```python
from build123d import *

# Parameters (mm, degrees)
MODEL_R             = 2.9
MODEL_R_2           = 3
MODEL_R_3           = 1.95
MODEL_R_4           = 4.665
MODEL_W             = 19.6
MODEL_H             = 4.75
BOSS_EXTRUDE1_DEPTH = 5.15


with BuildPart() as part:
    # Model → Boss-Extrude1 (new body)
    with BuildSketch(Plane.XY):
        with BuildLine():
            Line((43.819984585, 81.048439688), (48.280015415, 78.473439688))
            Line((48.280015415, 78.473439688), (57.214943747, 93.949189523))
            ThreePointArc((57.214943747, 93.949189523), (60.358438208, 91.961181686), (63.432925851, 89.868036131))
            Line((63.432925851, 89.868036131), (56.520818931, 77.895915758))
            Line((56.520818931, 77.895915758), (60.020818931, 71.833737931))
            Line((60.020818931, 71.833737931), (72.810336239, 79.217769192))
            Line((72.810336239, 79.217769192), (79.758802159, 67.182673184))
            ThreePointArc((79.758802159, 67.182673184), (87.004437854, 62.632864027), (87.321870319, 54.083054869))
            Line((87.321870319, 54.083054869), (92.810336239, 44.57675304))
            Line((92.810336239, 44.57675304), (80.020818931, 37.19272178))
            Line((80.020818931, 37.19272178), (95.720818931, 9.999524101))
            Line((95.720818931, 9.999524101), (109.544554943, 9.999524101))
            ThreePointArc((109.544554943, 9.999524101), (109.819966834, 6.290857214), (109.969856665, 2.575))
            Line((109.969856665, 2.575), (92.1, 2.575))
            Line((92.1, 2.575), (92.1, -2.575))
            Line((92.1, -2.575), (109.969856665, -2.575))
            ThreePointArc((109.969856665, -2.575), (109.819947856, -6.291188516), (109.544494609, -10.000185045))
            Line((109.544494609, -10.000185045), (95.720280769, -10.000185045))
            Line((95.720280769, -10.000185045), (56.520280769, -77.896576702))
            Line((56.520280769, -77.896576702), (63.432272389, -89.86849737))
            ThreePointArc((63.432272389, -89.86849737), (60.358103868, -91.961401128), (57.214943747, -93.949189523))
            Line((57.214943747, -93.949189523), (48.280015415, -78.473439688))
            Line((48.280015415, -78.473439688), (43.819984585, -81.048439688))
            Line((43.819984585, -81.048439688), (52.754912918, -96.524189523))
            ThreePointArc((52.754912918, -96.524189523), (49.461727838, -98.252417168), (46.112001713, -99.868329805))
            Line((46.112001713, -99.868329805), (39.2, -87.896391657))
            Line((39.2, -87.896391657), (32.2, -87.896391657))
            Line((32.2, -87.896391657), (32.2, -102.664454178))
            Line((32.2, -102.664454178), (18.303068161, -102.664454178))
            ThreePointArc((18.303068161, -102.664454178), (10.74, -106.664454178), (3.17693184, -102.664454178))
            Line((3.17693184, -102.664454178), (-7.8, -102.664454178))
            Line((-7.8, -102.664454178), (-7.8, -87.896391657))
            Line((-7.8, -87.896391657), (-39.2, -87.896391657))
            Line((-39.2, -87.896391657), (-46.112001713, -99.868329805))
            ThreePointArc((-46.112001713, -99.868329805), (-49.461727838, -98.252417168), (-52.754912918, -96.524189523))
            Line((-52.754912918, -96.524189523), (-43.819984585, -81.048439689))
            Line((-43.819984585, -81.048439689), (-48.280015415, -78.473439689))
            Line((-48.280015415, -78.473439689), (-57.214943747, -93.949189523))
            ThreePointArc((-57.214943747, -93.949189523), (-60.358012455, -91.961461126), (-63.432093724, -89.868623478))
            Line((-63.432093724, -89.868623478), (-56.52019722, -77.896867556))
            Line((-56.52019722, -77.896867556), (-60.02019722, -71.834689729))
            Line((-60.02019722, -71.834689729), (-72.809714528, -79.218720989))
            Line((-72.809714528, -79.218720989), (-79.758180447, -67.183624982))
            ThreePointArc((-79.758180447, -67.183624982), (-87.003816143, -62.633815824), (-87.321248608, -54.084006667))
            Line((-87.321248608, -54.084006667), (-92.809714528, -44.577704838))
            Line((-92.809714528, -44.577704838), (-80.02019722, -37.193673578))
            Line((-80.02019722, -37.193673578), (-95.72019722, -10.000475899))
            Line((-95.72019722, -10.000475899), (-109.544468057, -10.000475899))
            ThreePointArc((-109.544468057, -10.000475899), (-109.819939504, -6.291334309), (-109.969856665, -2.575))
            Line((-109.969856665, -2.575), (-92.1, -2.575))
            Line((-92.1, -2.575), (-92.1, 2.575))
            Line((-92.1, 2.575), (-109.969856665, 2.575))
            ThreePointArc((-109.969856665, 2.575), (-109.819958483, 6.291003006), (-109.544528393, 9.999814955))
            Line((-109.544528393, 9.999814955), (-95.720735382, 9.999814955))
            Line((-95.720735382, 9.999814955), (-56.520735382, 77.896206612))
            Line((-56.520735382, 77.896206612), (-63.432747187, 89.86816224))
            ThreePointArc((-63.432747187, 89.86816224), (-60.358346795, 91.961241684), (-57.214943747, 93.949189523))
            Line((-57.214943747, 93.949189523), (-48.280015415, 78.473439689))
            Line((-48.280015415, 78.473439689), (-43.819984585, 81.048439689))
            Line((-43.819984585, 81.048439689), (-52.754912918, 96.524189523))
            ThreePointArc((-52.754912918, 96.524189523), (-49.461727838, 98.252417168), (-46.112001713, 99.868329805))
            Line((-46.112001713, 99.868329805), (-39.2, 87.896391657))
            Line((-39.2, 87.896391657), (-32.2, 87.896391657))
            Line((-32.2, 87.896391657), (-32.2, 102.664454178))
            Line((-32.2, 102.664454178), (-18.30306816, 102.664454178))
            ThreePointArc((-18.30306816, 102.664454178), (-10.74, 106.664454178), (-3.176931839, 102.664454178))
            Line((-3.176931839, 102.664454178), (7.8, 102.664454178))
            Line((7.8, 102.664454178), (7.8, 87.896391657))
            Line((7.8, 87.896391657), (39.2, 87.896391657))
            Line((39.2, 87.896391657), (46.112001713, 99.868329805))
            ThreePointArc((46.112001713, 99.868329805), (49.461727838, 98.252417168), (52.754912918, 96.524189523))
            Line((52.754912918, 96.524189523), (43.819984585, 81.048439688))
        make_face()
        with Locations((-63, 0)):
            Circle(MODEL_R, mode=Mode.SUBTRACT)
        with Locations((-31.5, -54.559600438)):
            Circle(MODEL_R, mode=Mode.SUBTRACT)
        with Locations((31.5, -54.559600438)):
            Circle(MODEL_R, mode=Mode.SUBTRACT)
        with Locations((63, 0)):
            Circle(MODEL_R, mode=Mode.SUBTRACT)
        with Locations((31.5, 54.559600438)):
            Circle(MODEL_R, mode=Mode.SUBTRACT)
        with Locations((-31.5, 54.559600438)):
            Circle(MODEL_R_2, mode=Mode.SUBTRACT)
        with Locations((-79.079683698, -58.058815824)):
            Circle(MODEL_R_3, mode=Mode.SUBTRACT)
        with Locations((79.08030541, 58.057864027)):
            Circle(MODEL_R_3, mode=Mode.SUBTRACT)
        Circle(MODEL_R_4, mode=Mode.SUBTRACT)
        with Locations((-10.74, 97.514454178)):
            Circle(MODEL_R_3, mode=Mode.SUBTRACT)
        with Locations((10.74, -97.514454178)):
            Circle(MODEL_R_3, mode=Mode.SUBTRACT)
        Polygon((33.357314709, 18.17343612), (29.243694041, 15.79843612), (39.043694041, -1.175661794), (43.157314709, 1.199338206), align=None, mode=Mode.SUBTRACT)
        Polygon((32.417314709, -19.80156388), (28.303694041, -17.42656388), (18.503694041, -34.400661794), (22.617314709, -36.775661794), align=None, mode=Mode.SUBTRACT)
        with Locations((-10.74, -35.6)):
            Rectangle(MODEL_W, MODEL_H, mode=Mode.SUBTRACT)
        Polygon((-33.357314709, -18.17343612), (-29.243694041, -15.79843612), (-39.043694041, 1.175661794), (-43.157314709, -1.199338206), align=None, mode=Mode.SUBTRACT)
        Polygon((-32.417314709, 19.80156388), (-28.303694041, 17.42656388), (-18.503694041, 34.400661794), (-22.617314709, 36.775661794), align=None, mode=Mode.SUBTRACT)
        Polygon((36.982871141, 24.122696529), (38.982587357, 20.659086443), (43.096208025, 23.034086443), (41.096491809, 26.497696529), (79.288239187, 48.547712159), (69.488239187, 65.521810073), (31.296521386, 43.47181152), (30.75621053, 44.407594854), (26.642587357, 42.032593408), (28.642871141, 38.568000264), (25.222097867, 36.593015894), (33.562097867, 22.147712159), align=None, mode=Mode.SUBTRACT)
        Polygon((37.382587357, -23.430367735), (41.496208025, -25.805367735), (53.836208025, -4.431860769), (49.722587357, -2.056860769), align=None, mode=Mode.SUBTRACT)
        Polygon((2.4, -44.089454178), (-1.6, -44.089454178), (-1.6, -48.839454177), (2.4, -48.839454177), (2.4, -92.939454178), (22, -92.939454178), (22, -48.839454177), (23.08, -48.839454177), (23.08, -44.089454178), (19.08, -44.089454178), (19.08, -40.139454177), (2.4, -40.139454177), align=None, mode=Mode.SUBTRACT)
        Polygon((-36.982303573, -24.123679586), (-38.982587357, -20.659086443), (-43.096208025, -23.034086443), (-41.095924241, -26.498679586), (-79.287617476, -48.548663957), (-69.487617476, -65.522761871), (-31.295924241, -43.472777501), (-30.756208025, -44.407593408), (-26.642587357, -42.032593408), (-28.642303573, -38.568983322), (-25.221476156, -36.593967692), (-33.561476156, -22.148663957), align=None, mode=Mode.SUBTRACT)
        Polygon((-37.382587357, 23.430367735), (-41.496208025, 25.805367735), (-53.836208025, 4.431860769), (-49.722587357, 2.056860769), align=None, mode=Mode.SUBTRACT)
        with Locations((10.74, 35.6)):
            Rectangle(MODEL_W, MODEL_H, mode=Mode.SUBTRACT)
        Polygon((-2.4, 44.089454178), (1.6, 44.089454178), (1.6, 48.839454177), (-2.4, 48.839454177), (-2.4, 92.939454178), (-22, 92.939454178), (-22, 48.839454177), (-23.08, 48.839454177), (-23.08, 44.089454178), (-19.08, 44.089454178), (-19.08, 40.139454177), (-2.4, 40.139454177), align=None, mode=Mode.SUBTRACT)
    extrude(amount=BOSS_EXTRUDE1_DEPTH)


solid = part.part
```
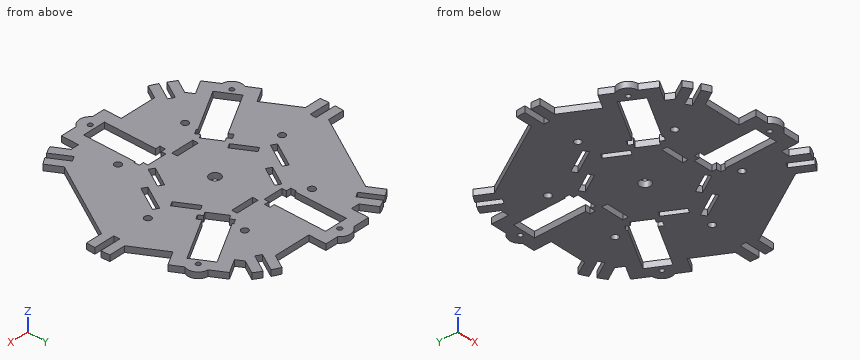
Verification items for the finished model (mm, model axes). Round coordinates to 2 decimals unless told otherwise and drop trailing zeros. Write each question's results on one line, items separated by ' | '. Start each with the question number.
1. Depth check by flat-ended pin: P1, Ø9.5, axis at x = -63, y = 0, coming from the -Z side; P2, Ø1, axis at y = -55, z = 2.5, coming from the -X side; P3, Ø2, axis at y = -43, z = 1.5, coming from the +X side; P4, Ø2.5, axis at x = -105.5, z = 3.5, coming from the +Y side. Enter the tip coordinate at first touch or a pass-through.
2. Material ranges on probe 1 along Y at (x, z) = (0, 0.5) (3 decimals); probe 2 along X at (y, z) = (-90, 2.6); probe 3 along Y at (x, z) = (59, 0.85), recorded low to high. Write a range as from..to.
3. Cross-section at A-A (z = 3.6). Count the separate pieces of the cut face and the enclosed holes in it, then the cut area to 3 significant figures.
Solutions:
1) P1: stops at z = 0 | P2: stops at x = -87.86 | P3: stops at x = 77.25 | P4: stops at y = 10
2) probe 1: y = -102.664..-48.839, -44.089..-4.665, 4.665..44.089, 48.839..102.664 | probe 2: x = -63.25..-54.93, -48.99..-40.41, -7.8..2.4, 22..32.2, 40.41..48.99, 54.93..63.25 | probe 3: y = -92.84..-82.19, -73.6..36.83, 59.47..73.6, 82.19..92.84
3) separate pieces: 1 | enclosed holes: 23 | area: 24,800 mm2
